Could you check a few things on this drawing? It's one solid part, dimensions in mm from its lowest x, y, z. A direction names the side the tool comes from. Round coordinates to 2 decimals unless told otherwise and drop trailing zeros. Write each loop counter-clockwise with the first axis right and the second up, starting at its lowest first coordinate (ties: lowest second). Pieces come first, ordered by that corner, then holes. Notation, with made-up numbers: M 75.25,2 L 107.25,2 A14 ccw 107.25,24 Z; hole C 22,28.25 d1. An arc over 180 degrees is marked long. One line per item, written item: value. Start each with the question number.
(1) I want a section at B-B on x = 9. Please give me the cut outline in (y, z), and give its area (3 significant figures).
(2) Thinking about a two-plate mould opening in Y: for the marked faces 1, 2, 3 and 4, which applies, released by +Y, released by -Y, zero draft, split by the parting line, or undercut?
(3) I want a section at A-A on y = 6.1. Please give me the cut outline in (x, z).
(4) I want a section at D-D on y = 10.25. Please give me the cut outline in (x, z), and give its area (3 significant figures).
(5) I'm going to push a flat-ended pin straight in: pin 1 Ø1.6 at (x, z) = (3.5, 4.5) entering from +Y. Where does the tip first touch, or does it pass through?
(6) I want a section at C-C on z = 5. Please give me the cut outline in (x, y).
(7) Which directions (+Z, -Z, +X, -X, +Y, -Y) give clear straight access to the entire face, cutting with the end or side of a thin tool? Please do the marked faces 5 and 6.
(8) If I drill on L1, parallel to Z at x = 3, y = 10; L2, parallel to X at y = 5, z = 5.5; L3, parallel to X at y = 4.75, z = 4.75, over which ranges is the centre line in solid material (lowest first)?
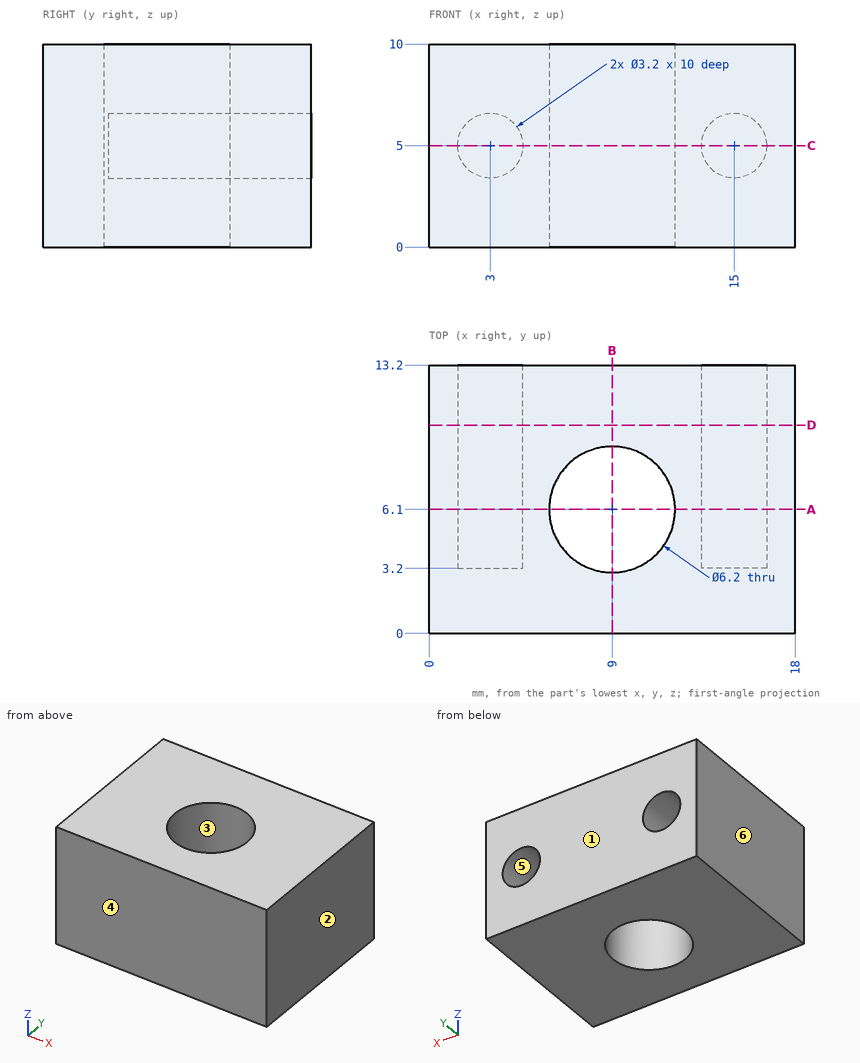
Found:
1. outline: M 0,0 L 3,0 L 3,10 L 0,10 Z; M 9.2,0 L 13.2,0 L 13.2,10 L 9.2,10 Z
1. area: 70.0 mm²
2. face 1: released by +Y
2. face 2: zero draft
2. face 3: undercut
2. face 4: released by -Y
3. outline: M 0,0 L 5.9,0 L 5.9,10 L 0,10 Z; M 12.1,0 L 18,0 L 18,10 L 12.1,10 Z; hole C 3,5 d3.2; hole C 15,5 d3.2
4. outline: M 0,0 L 18,0 L 18,10 L 0,10 Z; hole C 3,5 d3.2; hole C 15,5 d3.2
4. area: 164 mm²
5. pin 1: stops at y = 3.2
6. outline: M 0,0 L 18,0 L 18,13.2 L 16.6,13.2 L 16.6,3.2 L 13.4,3.2 L 13.4,13.2 L 4.6,13.2 L 4.6,3.2 L 1.4,3.2 L 1.4,13.2 L 0,13.2 Z; hole C 9,6.1 d6.2
7. face 5: +Y
7. face 6: +Z, -Z, -X, +Y, -Y
8. L1: z = 0 to 3.4, 6.6 to 10
8. L2: x = 0 to 1.48, 4.52 to 6.1, 11.9 to 13.48, 16.52 to 18
8. L3: x = 0 to 1.42, 4.58 to 6.21, 11.79 to 13.42, 16.58 to 18
